```python
from build123d import *

# Parameters (mm, degrees)
REVOLVE1_ANGLE      = 180
BOSS_EXTRUDE1_DEPTH = 70
SKETCH4_R           = 7.5
CUT_EXTRUDE1_DEPTH  = 9
SHELL1_DEPTH        = 61
SHELL1_START        = 61
SHELL1_2_DEPTH      = 8
SHELL1_3_ANGLE      = 180


with BuildPart() as part:
    # Sketch2 → Revolve1 (revolve)
    with BuildSketch(Plane.XY):
        with BuildLine():
            Line((0, 0), (0, 20))
            ThreePointArc((0, 20), (4.848310738, 18.582472089), (8.169373523, 14.776418441))
            Line((8.169373523, 14.776418441), (15, 0))
            Line((15, 0), (0, 0))
        make_face()
    revolve(axis=Axis((0, 0, 0), (0, 1, 0)), revolution_arc=REVOLVE1_ANGLE)

    # Sketch3 → Boss-Extrude1 (add)
    with BuildSketch(Plane.XY):
        with BuildLine():
            Line((-15, 0), (15, 0))
            Line((15, 0), (8.169373523, 14.776418441))
            ThreePointArc((8.169373523, 14.776418441), (0, 20), (-8.169373523, 14.776418441))
            Line((-8.169373523, 14.776418441), (-15, 0))
        make_face()
    extrude(amount=BOSS_EXTRUDE1_DEPTH)

    # Sketch4 → Cut-Extrude1 (cut)
    with BuildSketch(Plane.XY.offset(70)):
        with Locations((0, 11)):
            Circle(SKETCH4_R)
    extrude(amount=-CUT_EXTRUDE1_DEPTH, mode=Mode.SUBTRACT)

    # Shell1: read off the stored shape, not the designer's step
    # Shell1 outline → Shell1 (cut)
    with BuildSketch(Plane.XY):
        with BuildLine():
            Line((-13.898324336, 0), (13.898324336, 0))
            Line((13.898324336, 0), (7.261665354, 14.356816392))
            ThreePointArc((7.261665354, 14.356816392), (0, 19), (-7.261665354, 14.356816392))
            Line((-7.261665354, 14.356816392), (-13.898324336, 0))
        make_face()
    extrude(amount=SHELL1_DEPTH, mode=Mode.SUBTRACT)

    # Shell1 2 outline → Shell1 2 (cut)
    with BuildSketch(Plane.XY.offset(SHELL1_START)):
        with BuildLine():
            Line((-8.466880482, 11.74962317), (-13.898324336, 0))
            Line((-13.898324336, 0), (13.898324336, 0))
            Line((13.898324336, 0), (8.466880482, 11.74962317))
            ThreePointArc((8.466880482, 11.74962317), (0, 2.5), (-8.466880482, 11.74962317))
        make_face()
    extrude(amount=SHELL1_2_DEPTH, mode=Mode.SUBTRACT)

    # Shell1 3 outline → Shell1 3 (revolve, cut)
    with BuildSketch(Plane.XY):
        with BuildLine():
            Line((13.898324336, 0), (7.261665354, 14.356816392))
            ThreePointArc((7.261665354, 14.356816392), (4.309609545, 17.73997519), (0, 19))
            Line((0, 19), (0, 0))
            Line((0, 0), (13.898324336, 0))
        make_face()
    revolve(axis=Axis((0, 0, 0), (0, 1, 0)), revolution_arc=SHELL1_3_ANGLE, mode=Mode.SUBTRACT)


solid = part.part
```
Source: CAD feature listing. Evaluate the final solid. Frame: model axes, mm. A direction names the side the tool comes from. Coordinates: 2 decimals unless noted, no trailing zeros. Write each loop counter-clockwise with the first axis right and the second up, starting at its lowest first coordinate (ties: lowest second). Pieces come first, ordered by that corner, then holes. Notation, with made-up numbers: M 45.25,-23.75 L 95.25,-23.75 A13 cw 95.25,-1.75 Z; hole C 1,-10.5 d2. An arc over 180 degrees is marked long. Answer as a JSON object with one key per item and string values.
1. Cut plane A-A on x = 0. Output: boundary loops of the cut face in (y, z), plus the area to 3 significant figures.
Evaluation:
{"outline": "M 0,-15 L 14.78,-8.17 A9 ccw 20,0 L 20,70 L 18.5,70 L 18.5,61 L 19,61 L 19,0 A8 cw 14.36,-7.26 L 0,-13.9 Z; M 0,69 L 2.5,69 L 2.5,61 L 3.5,61 L 3.5,70 L 0,70 Z", "area": "112 mm^2"}
2. Cut plane D-D on y = 16. Output: boundary loops of the cut face in (x, z) (3 decimals), plus the area to 3 significant figures.
Evaluation:
{"outline": "M -7.483,0 A7.483 ccw 7.483,0 L 7.483,70 L 5.59,70 L 5.59,61 L 6.245,61 L 6.245,0 A6.245 cw -6.245,0 L -6.245,61 L -5.59,61 L -5.59,70 L -7.483,70 Z", "area": "212 mm^2"}
3. Cut plane C-C on y = 11. Output: boundary loops of the cut face in (x, z), plus the area to 3 significant figures.
Evaluation:
{"outline": "M -9.92,0 A9.92 ccw 9.92,0 L 9.92,70 L 7.5,70 L 7.5,61 L 8.5,61 L 8.5,69 L 8.81,69 L 8.81,0 A8.81 cw -8.81,0 L -8.81,69 L -8.5,69 L -8.5,61 L -7.5,61 L -7.5,70 L -9.92,70 Z", "area": "205 mm^2"}
4. Access query for faces 5 (the conical face through (0.24, 8.93, -10.87)), 6 (the flat face through (0, 3, 61)). Directions: +Z, -Z, +X, -X, +Y, -Y. A direction counts if a zero-diameter tool reaches every point of the face in a straight line with its end or side. Return the directions, or none.
Evaluation:
{"face 5": "-Z, +Y", "face 6": "-Y"}
5. Ray query, L1, parallel to Y at x = 0, z = 67.25; L2, parallel to X at y = 17.5, z = 41; L3, parallel to X at y = 15.75, z = 1.5. Return the intervals inside material, ascending.
Evaluation:
{"L1": "2.5 to 3.5, 18.5 to 20", "L2": "-6.22 to -4.66, 4.66 to 6.22", "L3": "-7.64 to -6.44, 6.44 to 7.64"}
6. Cut plane B-B on z = 41. Output: boundary loops of the cut face in (x, y).
Evaluation:
{"outline": "M -15,0 L -13.9,0 L -7.26,14.36 A8 cw 7.26,14.36 L 13.9,0 L 15,0 L 8.17,14.78 A9 ccw -8.17,14.78 Z"}
7. Draft query along X for faces 1 (the flat face through (14.4, 0, 24.2)), 2 (the flat face through (11.633, 7.285, 34.51)), 3 (the cylindrical face through (0, 20, 35)), 4 (the cylindrical face through (-1.63, 3.68, 65.56)). Return one class per face: released by +X, released by -X, zero draft, split by the parting line, or undercut.
Evaluation:
{"face 1": "zero draft", "face 2": "released by +X", "face 3": "split by the parting line", "face 4": "undercut"}
8. Contact query for flat-ended pins moving along their axis: P1, Ø10, axis at y = 8.5, z = -3.5, coming from the -X side; P2, Ø5, axis at x = -10.5, z = -3, coming from the +Y side; P3, Ø5, axis at y = 16, z = 36, coming from the +X side. Output: stop coordinate, or through.
Evaluation:
{"P1": "x = -13.12", "P2": "y = 14.23", "P3": "x = 8.76"}
